Here's how the part is built. I have some questions about the finished solid (model axes, mm). Face numbers are marked on the shaded views. A direction names the side the tool comes from. Round coordinates to 2 decimals unless told otherwise and drop trailing zeros. Order: outer loops, then holes, each group sorted by start corner. A loop starts at its lowest first (then second) coordinate and runs counter-clockwise, first axis right, second up. Notation, with made-up numbers: (22, -25.75) -> (63, -25.75) arc R24 ccw to (63, 3.25) -> close; hole circle Ø4 at (88, 89.5). An arc over 180 degrees is marked (long way). Use a Markdown table: item, result. Add a question column.
(1) I want a section at A-A, the plane z = 9. Please give me the cut outline in (x, y).
(2) Thinking about a two-plate mould opening in X: for the marked faces 3, 4 and 5, which applies, pulls with the +X half, pulls with the -X half, needs draft (parallel to the pull), parting line crosses it, or undercut?
(3) I'm going to push a flat-ended pin straight in: P1, Ø1.5, axis at x = 36, z = 3, coming from the +Y side. Where does the tip first touch, or does it pass through?
(4) I want a section at D-D, the plane z = 15. Please give me the cut outline in (x, y), then the cut area to 3 significant figures.
(5) I want a section at C-C, the plane y = -7.25. Please give me the cut outline in (x, z).
(6) I want a section at B-B, the plane x = 44. Please give me the cut outline in (y, z), then the cut area to 3 significant figures.
(7) On a 3-axis mill with a long thin cutter (end or side, diameter ignored), from which of +Z, -Z, +X, -X, +Y, -Y can I reach the whole of each face in a straight line? I mean the marked faces 1 and 2. Say none if no direction works.
(8) If I drill on probe 1 along Z at (x, y) = (44, -26.65); probe 2 along X at (y, z) = (-6, 8.5); probe 3 along X at (y, z) = (-18.25, 11.5), over which ranges is the centre line in solid material (lowest first)?
from build123d import *

# Parameters (mm, degrees)
F1_DEPTH = 18
F2_R     = 1.5
F3_DEPTH = 28.001
F4_SIZE2 = 4.5
F4_SIZE  = 8
F5_R     = 2


with BuildPart() as f1:
    # F0 (on Top) → F1 (new body)
    with BuildSketch(Plane.XY):
        Polygon((3, 0), (0, 0), (0, -28), (60, -28), (60, 0), (57, 0), (57, -25), (3, -25), align=None)
    extrude(amount=F1_DEPTH)

    # F2 (on face) → F3 (cut, through all)
    with BuildSketch(Plane.XZ.offset(28)):
        with Locations((44, 9)):
            Circle(F2_R)
    extrude(amount=-F3_DEPTH, mode=Mode.SUBTRACT)

    # F4
    f4_edges = [f1.edges().sort_by_distance(p)[0] for p in [
        (3, -25, 9),
    ]]
    f4_side = f1.faces().sort_by_distance((3, -12.5, 9))[0]
    chamfer(f4_edges, length=F4_SIZE, length2=F4_SIZE2, reference=f4_side)

    # F5
    f5_edges = [f1.edges().sort_by_distance(p)[0] for p in [
        (57, -25, 9),
        (7.5, -25, 9),
        (3, -17, 9),
        (3, 0, 9),
    ]]
    fillet(f5_edges, radius=F5_R)


solid = f1.part
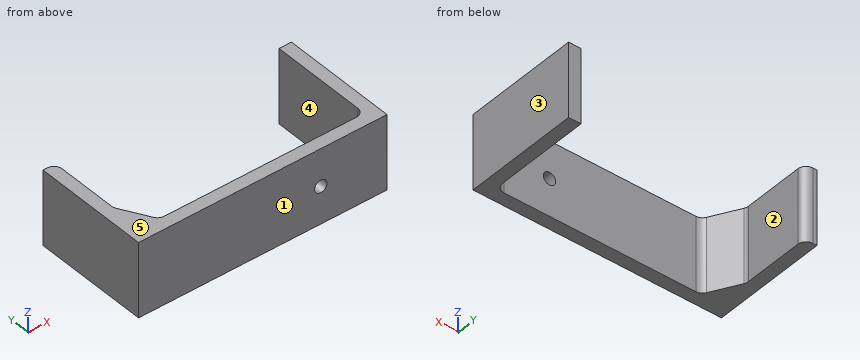
Taken from the geometry:
| question | item | result |
|---|---|---|
| 1 | outline | (0, -28) -> (42.5, -28) -> (42.5, -25) -> (8.67, -25) arc R2 cw to (6.93, -23.98) -> (3.26, -17.46) arc R2 cw to (3, -16.48) -> (3, -2) arc R2 ccw to (1, 0) -> (0, 0) -> close; (45.5, -28) -> (60, -28) -> (60, 0) -> (57, 0) -> (57, -23) arc R2 cw to (55, -25) -> (45.5, -25) -> close |
| 2 | face 3 | pulls with the +X half |
| 2 | face 4 | undercut |
| 2 | face 5 | needs draft |
| 3 | P1 | stops at y = -25 |
| 4 | outline | (0, -28) -> (60, -28) -> (60, 0) -> (57, 0) -> (57, -23) arc R2 cw to (55, -25) -> (8.67, -25) arc R2 cw to (6.93, -23.98) -> (3.26, -17.46) arc R2 cw to (3, -16.48) -> (3, -2) arc R2 ccw to (1, 0) -> (0, 0) -> close |
| 4 | area | 348 mm2 |
| 5 | outline | (0, 0) -> (3, 0) -> (3, 18) -> (0, 18) -> close; (57, 0) -> (60, 0) -> (60, 18) -> (57, 18) -> close |
| 6 | outline | (-28, 0) -> (-25, 0) -> (-25, 7.5) -> (-28, 7.5) -> close; (-28, 10.5) -> (-25, 10.5) -> (-25, 18) -> (-28, 18) -> close |
| 6 | area | 45.0 mm2 |
| 7 | face 1 | +Z, -Z, +X, -X, -Y |
| 7 | face 2 | +Z, -Z, +Y |
| 8 | probe 1 | z = 0 to 7.5, 10.5 to 18 |
| 8 | probe 2 | x = 0 to 3, 57 to 60 |
| 8 | probe 3 | x = 0 to 3.7, 57 to 60 |
